Drawing for the job (mm, zero at the part's lowest x, y, z). A direction names the side the tool comes from. Round coordinates to 2 decimals unless told otherwise and drop trailing zeros. Order: outer loops, then holes, each group sorted by start corner. A loop starts at its lowest first (then second) coordinate and runs counter-clockwise, first axis right, second up. Notation, with made-up numbers: M -19,54 L 19,54 A27 ccw 19,90 Z; hole C 38.25,-10.5 d8. An arc over 180 degrees is marked long. Answer as CSV lines item,"result". Start each with the question number.
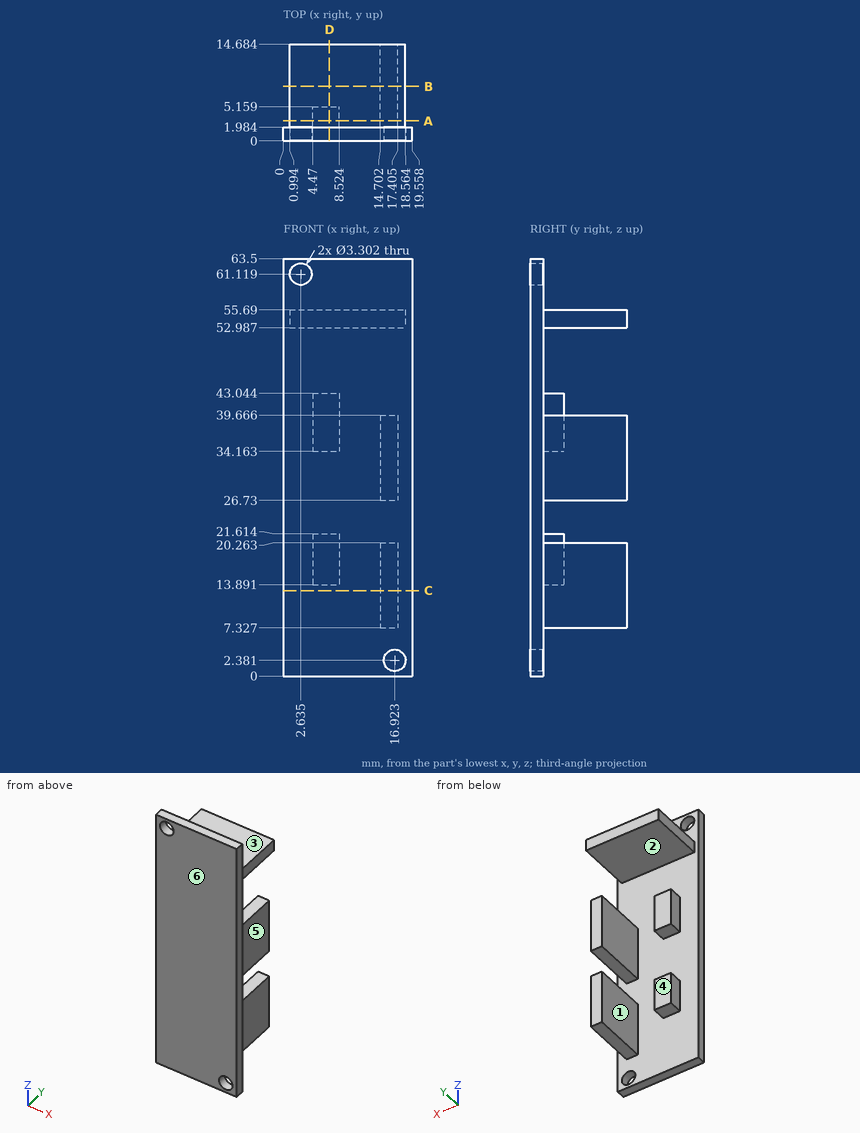
Q1. Band-saw the part on C-C, the plane z = 13. Write the cut outline in (x, y) (1 decimal).
Q2. Probe line 1 along Z through (x, y) = (17.25, 13.25) (1 decimal); line 2 along X through (y, z) = (4.25, 38.5) (1 decimal); line 3 along X through (y, z) = (9, 13) (1 decimal). List the from-to ranges inside material, lowest first. Write a range as from..to.
Q3. Tool access for the marked faces 4, 5 and 6: list every direction of +Z, -Z, +X, -X, +Y, -Y with a clear straight run to the whole face (end or side of a thin tool).
Q4. Mould opens along Z. For the marked faces 1, 2 and 3 say: +Z half, -Z half, draft (parallel to the pull), parting line (faces both ways), or undercut.
Q5. Drop flat-ended pins along their axis: P1, Ø3.5, axis at x = 7, y = 4, coming from the -Z side; P2, Ø3.5, axis at y = 4.5, z = 37.5, coming from the -X side; P3, Ø6.5, axis at y = 10.5, z = 16.5, coming from the -X side; P4, Ø4, axis at x = 8, z = 12, coming from the -Y side. Give the stop position or say it passes through.
Q6. Band-saw the part on A-A, the plane y = 3. Write the cut outline in (x, z) (1 decimal).
Q7. Band-saw the part on D-D, the plane x = 7. Write the cut outline in (y, z) (1 decimal).
Q8. Band-saw the part on B-B, the plane y = 8.25. Write the cut outline in (x, z) (1 decimal).
Answer:
1,outline,"M 0,0 L 19.6,0 L 19.6,2 L 17.4,2 L 17.4,14.7 L 14.7,14.7 L 14.7,2 L 0,2 Z"
2,line 1,"z = 7.3..20.3, 26.7..39.7, 53..55.7"
2,line 2,"x = 4.5..8.5, 14.7..17.4"
2,line 3,"x = 14.7..17.4"
3,face 4,"-Z, -X, +Y"
3,face 5,"-Z, +X, +Y"
3,face 6,"+Z, -Z, +X, -X, -Y"
4,face 1,"draft"
4,face 2,"undercut"
4,face 3,"+Z half"
5,P1,"stops at z = 13.89"
5,P2,"stops at x = 4.47"
5,P3,"stops at x = 14.7"
5,P4,"stops at y = 0"
6,outline,"M 1,53 L 18.6,53 L 18.6,55.7 L 1,55.7 Z; M 4.5,13.9 L 8.5,13.9 L 8.5,21.6 L 4.5,21.6 Z; M 4.5,34.2 L 8.5,34.2 L 8.5,43 L 4.5,43 Z; M 14.7,7.3 L 17.4,7.3 L 17.4,20.3 L 14.7,20.3 Z; M 14.7,26.7 L 17.4,26.7 L 17.4,39.7 L 14.7,39.7 Z"
7,outline,"M 0,0 L 2,0 L 2,13.9 L 5.2,13.9 L 5.2,21.6 L 2,21.6 L 2,34.2 L 5.2,34.2 L 5.2,43 L 2,43 L 2,53 L 14.7,53 L 14.7,55.7 L 2,55.7 L 2,63.5 L 0,63.5 Z"
8,outline,"M 1,53 L 18.6,53 L 18.6,55.7 L 1,55.7 Z; M 14.7,7.3 L 17.4,7.3 L 17.4,20.3 L 14.7,20.3 Z; M 14.7,26.7 L 17.4,26.7 L 17.4,39.7 L 14.7,39.7 Z"
